```python
from build123d import *

# Parameters (mm, degrees)
BOSS_EXTRUDE1_DEPTH      = 25
BOSS_EXTRUDE1_DEPTH_BACK = 25
SKETCH2_W                = 30
SKETCH2_H                = 40
CUT_EXTRUDE1_DEPTH       = 96.524865873
BOSS_EXTRUDE2_REACH      = 90.318
SKETCH3_R                = 12.5
STRUCTURAL_MEMBER1_DEPTH = 200
BOSS_EXTRUDE3_DEPTH      = 10
BOSS_EXTRUDE4_DEPTH      = 50
BOSS_EXTRUDE4_DEPTH_BACK = 10
CUT_EXTRUDE6_START       = -30
CUT_EXTRUDE6_DEPTH       = 30
SKETCH16_R               = 12.5
CUT_EXTRUDE7_DEPTH       = 325.384031666
FILLET1_R                = 10
FILLET2_R                = 2
FILLET3_R                = 2
SKETCH19_W               = 30
SKETCH19_H               = 10
BOSS_EXTRUDE6_DEPTH      = 20
FILLET5_R                = 15
CUT_EXTRUDE8_REACH       = 328.075
SKETCH20_R               = 5
FILLET5_OF_MIRROR9_R     = 15
LPATTERN1_START          = -5
LPATTERN1_OUTLINE_R      = 5
LPATTERN1_DEPTH          = 10
CUT_EXTRUDE9_START       = 35
CUT_EXTRUDE9_OUTLINE_W   = 30
CUT_EXTRUDE9_OUTLINE_H   = 10
CUT_EXTRUDE9_DEPTH       = 20
CUT_EXTRUDE10_START      = -25
CUT_EXTRUDE10_OUTLINE_R  = 5
CUT_EXTRUDE10_DEPTH      = 10


# Read off the part's stored shape, not the designer's step: Cut-Extrude6, LPattern1, Cut-Extrude9, Cut-Extrude10
# Some blends are built 0.0001 mm under size
with BuildPart() as part:
    # Sketch1 → Boss-Extrude1 (new, two sides: drawn at the far end of the back side and taken through both)
    with BuildSketch(Plane.XY.offset(-BOSS_EXTRUDE1_DEPTH_BACK)):
        with BuildLine():
            Line((0, 20), (70, 20))
            Line((70, 20), (70, -20))
            Line((70, -20), (0, -20))
            ThreePointArc((0, -20), (-20, 0), (0, 20))
        make_face()
    extrude(amount=BOSS_EXTRUDE1_DEPTH + BOSS_EXTRUDE1_DEPTH_BACK)

    # Sketch2 → Cut-Extrude1 (cut, through all)
    with BuildSketch(Plane(origin=(70, 0, 0), x_dir=(0, 0, -1), z_dir=(1, 0, 0))):
        Rectangle(SKETCH2_W, SKETCH2_H)
    extrude(amount=-CUT_EXTRUDE1_DEPTH, mode=Mode.SUBTRACT)


with BuildPart() as cut_extrude1_piece_1:
    # of the separate pieces the step leaves, piece 1, a body of its own (cut_extrude1_pieces)
    add(part.part.solids().sort_by_distance((0, 20, -25))[0])

    # Sketch3 → Boss-Extrude2 (add, up to next)
    with BuildSketch(Plane.XY.offset(25), mode=Mode.PRIVATE) as boss_extrude2_sk1:
        Circle(SKETCH3_R)
    boss_extrude2_tool1 = extrude(boss_extrude2_sk1.sketch, amount=-BOSS_EXTRUDE2_REACH, mode=Mode.PRIVATE) - cut_extrude1_piece_1.part


with BuildPart() as cut_extrude1_piece_2:
    # of the separate pieces the step leaves, piece 2, a body of its own (cut_extrude1_pieces)
    add(part.part.solids().sort_by_distance((0, 20, 15))[0])


with BuildPart() as cut_extrude1_piece_1_1:
    add(cut_extrude1_piece_1.part)

    add(cut_extrude1_piece_2.part)  # Boss-Extrude2 merges Cut-Extrude1 piece 2
    add(boss_extrude2_tool1.solids().sort_by_distance((0, 0, 25))[0])



with BuildPart() as body_2:
    # Sketch11 → Structural Member1 (new body)
    with BuildSketch(Plane(origin=(70, 0, 0), x_dir=(0, 0, 1), z_dir=(1, 0, 0))):
        with BuildLine():
            Line((-10, -35), (10, -35))
            ThreePointArc((10, -35), (17.071067812, -32.071067812), (20, -25))
            Line((20, -25), (20, 25))
            ThreePointArc((20, 25), (17.071067812, 32.071067812), (10, 35))
            Line((10, 35), (-10, 35))
            ThreePointArc((-10, 35), (-17.071067812, 32.071067812), (-20, 25))
            Line((-20, 25), (-20, -25))
            ThreePointArc((-20, -25), (-17.071067812, -32.071067812), (-10, -35))
        make_face()
        with BuildLine():
            Line((-10, -30), (10, -30))
            ThreePointArc((10, -30), (13.535533906, -28.535533906), (15, -25))
            Line((15, -25), (15, 25))
            ThreePointArc((15, 25), (13.535533906, 28.535533906), (10, 30))
            Line((10, 30), (-10, 30))
            ThreePointArc((-10, 30), (-13.535533906, 28.535533906), (-15, 25))
            Line((-15, 25), (-15, -25))
            ThreePointArc((-15, -25), (-13.535533906, -28.535533906), (-10, -30))
        make_face(mode=Mode.SUBTRACT)
    extrude(amount=STRUCTURAL_MEMBER1_DEPTH)


with BuildPart() as cut_extrude1_piece_1_2:
    add(cut_extrude1_piece_1_1.part)

    add(body_2.part)  # Boss-Extrude3 merges body 2
    # Sketch12 → Boss-Extrude3 (add)
    with BuildSketch(Plane.ZY.offset(-70)):
        with BuildLine():
            Line((20, -25), (20, 25))
            ThreePointArc((20, 25), (17.071067812, 32.071067812), (10, 35))
            Line((10, 35), (-10, 35))
            ThreePointArc((-10, 35), (-17.071067812, 32.071067812), (-20, 25))
            Line((-20, 25), (-20, -25))
            ThreePointArc((-20, -25), (-17.071067812, -32.071067812), (-10, -35))
            Line((-10, -35), (10, -35))
            ThreePointArc((10, -35), (17.071067812, -32.071067812), (20, -25))
        make_face()
    extrude(amount=BOSS_EXTRUDE3_DEPTH)

    # Sketch14 → Boss-Extrude4 (add, two sides: drawn at the far end of the back side and taken through both)
    with BuildSketch(Plane(origin=(270, 0, 0), x_dir=(0, 0, -1), z_dir=(1, 0, 0)).offset(-BOSS_EXTRUDE4_DEPTH_BACK)):
        with BuildLine():
            Line((15, -25), (15, 25))
            ThreePointArc((15, 25), (13.535533906, 28.535533906), (10, 30))
            Line((10, 30), (-10, 30))
            ThreePointArc((-10, 30), (-13.535533906, 28.535533906), (-15, 25))
            Line((-15, 25), (-15, -25))
            ThreePointArc((-15, -25), (-13.535533906, -28.535533906), (-10, -30))
            Line((-10, -30), (10, -30))
            ThreePointArc((10, -30), (13.535533906, -28.535533906), (15, -25))
        make_face()
    extrude(amount=BOSS_EXTRUDE4_DEPTH + BOSS_EXTRUDE4_DEPTH_BACK)

    # Cut-Extrude6 outline → Cut-Extrude6 (cut)
    with BuildSketch(Plane.XY.offset(15).offset(CUT_EXTRUDE6_START)):
        with BuildLine():
            Line((270, -25), (270, -30))
            Line((270, -30), (320, -30))
            Line((320, -30), (320, -2.73e-07))
            ThreePointArc((320, -2.73e-07), (312.677669433, -17.677669626), (295, -25))
            Line((295, -25), (270, -25))
        make_face()
        with BuildLine():
            Line((270, 30), (270, 25))
            Line((270, 25), (295, 25))
            ThreePointArc((295, 25), (312.677669626, 17.677669433), (320, -2.73e-07))
            Line((320, -2.73e-07), (320, 30))
            Line((320, 30), (270, 30))
        make_face()
    extrude(amount=CUT_EXTRUDE6_DEPTH, mode=Mode.SUBTRACT)

    # Sketch16 → Cut-Extrude7 (cut, through all)
    with BuildSketch(Plane.XY.offset(15)):
        with Locations((295, 0)):
            Circle(SKETCH16_R)
    extrude(amount=-CUT_EXTRUDE7_DEPTH, mode=Mode.SUBTRACT)

    # Fillet1
    # the kernel refuses this fillet: 10 mm, written as the material it takes off along each edge
    with BuildSketch(Plane(origin=(70, 41.650635095, -25), x_dir=(0, 0, 1), z_dir=(0, -1, 0))) as fillet1_piece_1:
        with BuildLine():
            CenterArc((10, 8.660254038), FILLET1_R, 180, 60)
            Line((0, 8.660254038), (-0.2, 8.660254038))
            Line((-0.2, 8.660254038), (-0.2, 0))
            Line((-0.2, 0), (0, -0.2))
            ThreePointArc((0, -0.2), (2.5, -0.2), (4.9, -0.173205081))
            Line((4.9, -0.173205081), (5, 0))
        make_face()
    extrude(amount=83.301270189, mode=Mode.SUBTRACT)
    with BuildSketch(Plane(origin=(70, 41.650635095, 25), x_dir=(0, 0, -1), z_dir=(0, -1, 0))) as fillet1_piece_2:
        with BuildLine():
            CenterArc((10, -8.660254038), FILLET1_R, 120, 60)
            Line((0, -8.660254038), (-0.2, -8.660254038))
            Line((-0.2, -8.660254038), (-0.2, 0))
            Line((-0.2, 0), (0, 0.2))
            ThreePointArc((0, 0.2), (2.5, 0.2), (4.9, 0.173205081))
            Line((4.9, 0.173205081), (5, 0))
        make_face()
    extrude(amount=83.301270189, mode=Mode.SUBTRACT)

    # Fillet2
    fillet2_edges = [cut_extrude1_piece_1_2.edges().sort_by_distance(p)[0] for p in [
        (-12.5, 0, 15),
        (30, 20, -15),
        (-20, 0, -15),
        (30, -20, -15),
        (-20, 0, 15),
        (30, 20, 15),
        (60, 0, -15),
        (30, -20, 15),
        (60, 0, 15),
        (60, 20, 17.5),
        (60, 20, -17.5),
        (60, -20, -17.5),
        (60, -20, 17.5),
    ]]
    fillet(fillet2_edges, radius=FILLET2_R)

    # Fillet3
    fillet3_edges = [cut_extrude1_piece_1_2.edges().sort_by_distance(p)[0] for p in [
        (66.339745962, 20, 23.660254038),
        (30.669872981, 20, 25),
        (-20, 0, 25),
        (66.339745962, -20, 23.660254038),
        (66.339745962, 20, -23.660254038),
        (30.669872981, 20, -25),
        (-20, 0, -25),
        (66.339745962, -20, -23.660254038),
        (30.669872981, -20, 25),
        (30.669872981, -20, -25),
    ]]
    fillet(fillet3_edges, radius=FILLET3_R)

    # Sketch19 → Boss-Extrude6 (add)
    with BuildSketch(Plane.XZ.offset(35)):
        with Locations((110, 0)):
            Rectangle(SKETCH19_W, SKETCH19_H)
    boss_extrude6 = extrude(amount=BOSS_EXTRUDE6_DEPTH)

    # Fillet5
    fillet5_edges = [cut_extrude1_piece_1_2.edges().sort_by_distance(p)[0] for p in [
        (95, -55, 0),
        (125, -55, 0),
    ]]
    fillet(fillet5_edges, radius=FILLET5_R - 0.0001)  # a hair under: the kernel refuses the full size

    # Sketch20 → Cut-Extrude8 (cut, up to next)
    with BuildSketch(Plane.XY.offset(5), mode=Mode.PRIVATE) as cut_extrude8_sk1:
        with Locations((110, -45)):
            Circle(SKETCH20_R)
    cut_extrude8_tool1 = extrude(cut_extrude8_sk1.sketch, amount=-CUT_EXTRUDE8_REACH, mode=Mode.PRIVATE) & cut_extrude1_piece_1_2.part
    cut_extrude8 = cut_extrude8_tool1.solids().sort_by_distance((110, -45, 5))[0]
    add(cut_extrude8, mode=Mode.SUBTRACT)

    # Mirror9: Boss-Extrude6, Cut-Extrude8 across plane
    add(boss_extrude6.mirror(Plane.ZX))
    add(cut_extrude8.mirror(Plane.ZX), mode=Mode.SUBTRACT)

    # Fillet5 of Mirror9
    fillet5_of_mirror9_edges = [cut_extrude1_piece_1_2.edges().sort_by_distance(p)[0] for p in [
        (95, 55, 0),
        (125, 55, 0),
    ]]
    fillet(fillet5_of_mirror9_edges, radius=FILLET5_OF_MIRROR9_R - 0.0001)  # a hair under: the kernel refuses the full size

    # LPattern1 outline → LPattern1 (add)
    # profile 1 of 2: a face of its own
    with BuildSketch(Plane.XY.offset(LPATTERN1_START)):
        with BuildLine():
            Line((195, 35), (225, 35))
            Line((225, 35), (225, 40))
            ThreePointArc((225, 40), (220.606601718, 50.606601718), (210, 55))
            ThreePointArc((210, 55), (199.393398282, 50.606601718), (195, 40))
            Line((195, 40), (195, 35))
        make_face()
        with Locations((210, 45)):
            Circle(LPATTERN1_OUTLINE_R, mode=Mode.SUBTRACT)
    # profile 2 of 2: a face of its own
    with BuildSketch(Plane.XY.offset(LPATTERN1_START)):
        with BuildLine():
            Line((225, -40), (225, -35))
            Line((225, -35), (195, -35))
            Line((195, -35), (195, -40))
            ThreePointArc((195, -40), (199.393398282, -50.606601718), (210, -55))
            ThreePointArc((210, -55), (220.606601718, -50.606601718), (225, -40))
        make_face()
        with Locations((210, -45)):
            Circle(LPATTERN1_OUTLINE_R, mode=Mode.SUBTRACT)
    extrude(amount=LPATTERN1_DEPTH)

    # Cut-Extrude9 outline → Cut-Extrude9 (cut)
    with BuildSketch(Plane(origin=(0, 0, 0), x_dir=(1, 0, 0), z_dir=(0, 1, 0)).offset(CUT_EXTRUDE9_START)):
        with Locations((110, 0)):
            Rectangle(CUT_EXTRUDE9_OUTLINE_W, CUT_EXTRUDE9_OUTLINE_H)
    extrude(amount=CUT_EXTRUDE9_DEPTH, mode=Mode.SUBTRACT)

    # Cut-Extrude10 outline → Cut-Extrude10 (cut)
    with BuildSketch(Plane.XY.offset(20).offset(CUT_EXTRUDE10_START)):
        with BuildLine():
            Line((225, -40), (225, -35))
            Line((225, -35), (195, -35))
            Line((195, -35), (195, -40))
            ThreePointArc((195, -40), (199.393398282, -50.606601718), (210, -55))
            ThreePointArc((210, -55), (220.606601718, -50.606601718), (225, -40))
        make_face()
        with Locations((210, -45)):
            Circle(CUT_EXTRUDE10_OUTLINE_R, mode=Mode.SUBTRACT)
    extrude(amount=CUT_EXTRUDE10_DEPTH, mode=Mode.SUBTRACT)


solid = cut_extrude1_piece_1_2.part
```
The model under review builds one solid part; all positions refer to its coordinate system, in mm. A direction names the side the tool comes from. Coordinates: 2 decimals unless noted, no trailing zeros. Write each loop counter-clockwise with the first axis right and the second up, starting at its lowest first coordinate (ties: lowest second). Pieces come first, ordered by that corner, then holes.
1) Machinability: for faces 4 (the face through (283, -25, 0)), 5 (the face through (164, 30, 0)), 6 (the face through (213.1, 40.7, 5)), which of the approach directions +Z, -Z, +X, -X, +Y, -Y give a long, thin tool a straight path to every point of the face, cutting with its end or side? Answer none if there is none.
2) We need section C-C on y = -45. State the section outline as (x, z) points, then the cut area to 3 significant figures.
3) The part is to be moulded in two halves that separate along Z. For faces 1 (the face through (166, -35, 0)), 2 (the face through (260, 0, 0)), 3 (the face through (21, 0, 25)), say which applies: pulls with the +Z half, pulls with the -Z half, needs draft (parallel to the pull), parting line crosses it, or undercut.
4) We need section A-A on z = 2. Count the separate pieces of the cut face and the enclosed holes in it, then the cut area to 3 significant figures.
5) We need section B-B on x = 231.5. State the section outline as (y, z) points.
6) Clearance check with flat-ended pins moving along their axes: pin 1 Ø1.5 at (x, y) = (88, -31.5) entering from -Z; pin 2 Ø25 at (x, y) = (298, 2.5) entering from -Z; pin 3 Ø15 at (x, y) = (206.5, -7) entering from +Z. State where each tip first meets the part, or that it passes through.
7) To check wall thickness, follow probe 1 along Z at (x, y) = (181.5, 20); probe 2 along Y at (x, z) = (110, 2); probe 3 along X at (y, z) = (26, 10.5). State the ranges of each line that lie inside material, in increasing order.
Answer list:
1. face 4: +Z, -Z, +X, -Y
1. face 5: none
1. face 6: +Z, +X, -X, +Y
2. outline: (95.86, -5) - (105, -5) - (105, 5) - (95.86, 5) - close; (115, -5) - (124.14, -5) - (124.14, 5) - (115, 5) - close
2. area: 183 mm2
3. face 1: needs draft
3. face 2: undercut
3. face 3: pulls with the +Z half
4. separate pieces: 2
4. enclosed holes: 4
4. area: 6,380 mm2
5. outline: (-35, -10) arc R10 ccw to (-25, -20) - (25, -20) arc R10 ccw to (35, -10) - (35, 10) arc R10 ccw to (25, 20) - (-25, 20) arc R10 ccw to (-35, 10) - close; hole (-30, -10) arc R5 ccw to (-25, -15) - (25, -15) arc R5 ccw to (30, -10) - (30, 10) arc R5 ccw to (25, 15) - (-25, 15) arc R5 ccw to (-30, 10) - close
6. pin 1: stops at z = -18.18
6. pin 2: stops at z = -15
6. pin 3: stops at z = 20
7. probe 1: z = -20 to -15, 15 to 20
7. probe 2: y = -55 to -50, -40 to -30, 30 to 35
7. probe 3: x = 60 to 70, 260 to 270
